Model file for the job. Use its own axes, mm. A direction names the side the tool comes from. Give positions to 0.01 mm unless a question says otherwise; leave off trailing zeros. Order: outer loops, then holes, each group sorted by start corner. A loop starts at its lowest first (then second) coordinate and runs counter-clockwise, first axis right, second up. Notation, with made-up numbers: (-15, 22) - (13, 22) arc R19 cw to (13, 37) - close; hole circle Ø10 at (35.5, 79). An arc over 180 degrees is marked (long way). Return JSON: item names as keys, results as strings. Group by question number.
from build123d import *

# Parameters (mm, degrees)
SKETCH1_R       = 1.6
BASE_DEPTH      = 23
BASE_DEPTH_BACK = 0.0001


with BuildPart() as part:
    # Sketch1 → Base (new body, two sides)
    with BuildSketch(Plane(origin=(0, 0, 0), x_dir=(1, 0, 0), z_dir=(0, 1, 0))) as base_sk:
        Polygon((-16, -7.499999998), (-7.5, -15.999999998), (7.5, -15.999999998), (16, -7.499999998), (16, 7.500000002), (11, 12.500000002), (11, 20.000000005), (12, 21.000000005), (17.500000004, 21.000000005), (21, 17.500000009), (21, -17.499999998), (17.5, -20.999999998), (-17.5, -20.999999998), (-21, -17.499999998), (-21, 17.500000009), (-17.500000004, 21.000000005), (-12, 21.000000005), (-11, 20.000000005), (-11, 12.500000002), (-16, 7.500000002), align=None)
        with Locations((-15.500000002, 15.5)):
            Circle(SKETCH1_R, mode=Mode.SUBTRACT)
        with Locations((-15.500000002, -15.5)):
            Circle(SKETCH1_R, mode=Mode.SUBTRACT)
        with Locations((15.500000002, -15.5)):
            Circle(SKETCH1_R, mode=Mode.SUBTRACT)
        with Locations((15.500000002, 15.5)):
            Circle(SKETCH1_R, mode=Mode.SUBTRACT)
    extrude(amount=BASE_DEPTH)
    extrude(base_sk.sketch, amount=-BASE_DEPTH_BACK)


solid = part.part
(1) Drill centre lines: L1, parallel to X at y = 14.5, z = -15.5; L2, parallel to X at y = 15.75, z = -3; L3, parallel to Z at x = 15.5, y = 7.25. Where is each one in solid material? Low to high.
(2) Pull direction X, two halves, no side cores. Call faces 1 (the face through (19.2, 11.7, -19.3)), 2 (the face through (-21, 12, 0)), 3 (the face through (15, 12, -21)), 4 (the face through (-11.5, 11.7, -20.5)): released by +X, released by -X, zero draft, split by the parting line, or undercut.
(3) Slice it at C-C (y = 10.25). Give the cut face in (x, z), and give its area (3 significant figures).
(4) Slice it at A-A (z = -15.5). Give the cut face in (x, y), and give its area (3 significant figures).
(5) 3-axis set-ups, long thin cutter, end or side, ignore diameter. For faces 5 (the face through (-13.5, 11.7, -10)), 6 (the face through (-19.2, 11.7, 19.3)), 7 (the face through (11, 12, -16)): which of +Z, -Z, +X, -X, +Y, -Y reach the whole face in a straight line?
(6) Drop flat-ended pins along their axis: pin 1 Ø1.9 at (x, z) = (-15.5, -15.5) entering from -Y; pin 2 Ø7.5 at (x, y) = (2.5, 6) entering from -Z; pin 3 Ø8 at (x, z) = (11.5, 10.5) entering from -Y. Give the stop position or say it passes through.
(7) Slice it at D-D (x = -2). Give the cut face in (y, z).
(8) Slice it at B-B (z = 8.5). Give the cut face in (x, y).
Result set:
{
 "1": {"L1": "x = -21 to -17.1, -13.9 to -11, 11 to 13.9, 17.1 to 21", "L2": "x = -21 to -16, 16 to 21", "L3": "z = -21 to -17.1, -13.9 to -8, 8 to 13.9, 17.1 to 21"},
 "2": {"face 1": "released by +X", "face 2": "released by -X", "face 3": "zero draft", "face 4": "undercut"},
 "3": {"outline": "(-21, -17.5) - (-17.5, -21) - (-12, -21) - (-11, -20) - (-11, -12.5) - (-16, -7.5) - (-16, 7.5) - (-7.5, 16) - (7.5, 16) - (16, 7.5) - (16, -7.5) - (11, -12.5) - (11, -20) - (12, -21) - (17.5, -21) - (21, -17.5) - (21, 17.5) - (17.5, 21) - (-17.5, 21) - (-21, 17.5) - close; hole circle Ø3.2 at (-15.5, -15.5); hole circle Ø3.2 at (-15.5, 15.5); hole circle Ø3.2 at (15.5, -15.5); hole circle Ø3.2 at (15.5, 15.5)", "area": "705 mm²"},
 "4": {"outline": "(-21, 0) - (-17.1, 0) - (-17.1, 23) - (-21, 23) - close; (-13.9, 0) - (-11, 0) - (-11, 23) - (-13.9, 23) - close; (11, 0) - (13.9, 0) - (13.9, 23) - (11, 23) - close; (17.1, 0) - (21, 0) - (21, 23) - (17.1, 23) - close", "area": "313 mm²"},
 "5": {"face 5": "+Y, -Y", "face 6": "+Z, -X, +Y, -Y", "face 7": "-Z, +Y, -Y"},
 "6": {"pin 1": "passes through", "pin 2": "stops at z = 16", "pin 3": "stops at y = 0"},
 "7": {"outline": "(0, 16) - (23, 16) - (23, 21) - (0, 21) - close"},
 "8": {"outline": "(-21, 0) - (-15, 0) - (-15, 23) - (-21, 23) - close; (15, 0) - (21, 0) - (21, 23) - (15, 23) - close"}
}
